```python
from build123d import *

# Parameters (mm, degrees)
SKETCH4_W                = 48.4
SKETCH4_H                = 35.4
BOTTOM_PLATE_DEPTH       = 3
SKETCH5_W                = 48.4
SKETCH5_H                = 3
SKETCH5_H_2              = 3.111627182
SIDE_PLATE_DEPTH         = 32.4
SKETCH6_W                = 48.4
SKETCH6_H                = 3
TOP_PLATE_1_DEPTH        = 6
SKETCH7_W                = 48.4
SKETCH7_H                = 3
TOP_PLATE_2_DEPTH        = 6
CAMERA_SCREW_HOLES_REACH = 64.688
SKETCH8_R                = 1
SKETCH10_R               = 1
CASE_ATTACHMENT_1_DEPTH  = 3
SKETCH10_4_R             = 1
CASE_ATTACHMENT_2_DEPTH  = 3


with BuildPart() as part:
    # Sketch4 → Bottom_Plate (new body)
    with BuildSketch(Plane.XY):
        with Locations((-19.226323529, -13.831389527)):
            Rectangle(SKETCH4_W, SKETCH4_H)
    extrude(amount=BOTTOM_PLATE_DEPTH)

    # Sketch5 → Side_Plate (add)
    with BuildSketch(Plane.XY.offset(3)):
        with Locations((-19.226323529, 2.368610473)):
            Rectangle(SKETCH5_W, SKETCH5_H)
        with Locations((-19.226323529, -29.975575936)):
            Rectangle(SKETCH5_W, SKETCH5_H_2)
    extrude(amount=SIDE_PLATE_DEPTH)

    # Sketch6 → Top_Plate_1 (add)
    with BuildSketch(Plane.XZ.offset(-0.868610473)):
        with Locations((-19.226323529, 33.9)):
            Rectangle(SKETCH6_W, SKETCH6_H)
    extrude(amount=TOP_PLATE_1_DEPTH)

    # Sketch7 → Top_Plate_2 (add)
    with BuildSketch(Plane(origin=(0, -28.419762345, 0), x_dir=(1, 0, 0), z_dir=(0, 1, 0))):
        with Locations((-19.226323529, -33.9)):
            Rectangle(SKETCH7_W, SKETCH7_H)
    extrude(amount=TOP_PLATE_2_DEPTH)

    # Sketch8 → Camera_Screw_Holes (cut, up to next)
    with BuildSketch(Plane.XY.offset(3), mode=Mode.PRIVATE) as camera_screw_holes_sk1:
        with Locations((-34.526323529, -19.719762345)):
            Circle(SKETCH8_R)
    camera_screw_holes_tool1 = extrude(camera_screw_holes_sk1.sketch, amount=-CAMERA_SCREW_HOLES_REACH, mode=Mode.PRIVATE) & part.part
    # Sketch8 → Camera_Screw_Holes (cut, up to next)
    with BuildSketch(Plane.XY.offset(3), mode=Mode.PRIVATE) as camera_screw_holes_sk2:
        with Locations((-34.611878154, -7.831372789)):
            Circle(SKETCH8_R)
    camera_screw_holes_tool2 = extrude(camera_screw_holes_sk2.sketch, amount=-CAMERA_SCREW_HOLES_REACH, mode=Mode.PRIVATE) & part.part
    # Sketch8 → Camera_Screw_Holes (cut, up to next)
    with BuildSketch(Plane.XY.offset(3), mode=Mode.PRIVATE) as camera_screw_holes_sk3:
        with Locations((-12.611878575, -7.835676936)):
            Circle(SKETCH8_R)
    camera_screw_holes_tool3 = extrude(camera_screw_holes_sk3.sketch, amount=-CAMERA_SCREW_HOLES_REACH, mode=Mode.PRIVATE) & part.part
    # Sketch8 → Camera_Screw_Holes (cut, up to next)
    with BuildSketch(Plane.XY.offset(3), mode=Mode.PRIVATE) as camera_screw_holes_sk4:
        with Locations((-12.526323529, -19.719762345)):
            Circle(SKETCH8_R)
    camera_screw_holes_tool4 = extrude(camera_screw_holes_sk4.sketch, amount=-CAMERA_SCREW_HOLES_REACH, mode=Mode.PRIVATE) & part.part
    add(camera_screw_holes_tool1.solids().sort_by_distance((-34.526324, -19.719762, 3))[0], mode=Mode.SUBTRACT)
    add(camera_screw_holes_tool2.solids().sort_by_distance((-34.611878, -7.831373, 3))[0], mode=Mode.SUBTRACT)
    add(camera_screw_holes_tool3.solids().sort_by_distance((-12.611879, -7.835677, 3))[0], mode=Mode.SUBTRACT)
    add(camera_screw_holes_tool4.solids().sort_by_distance((-12.526324, -19.719762, 3))[0], mode=Mode.SUBTRACT)

    # Sketch10 → Case_Attachment_1 (add)
    with BuildSketch(Plane(origin=(0, 0, 0), x_dir=(-1, 0, 0), z_dir=(0, 0, -1))):
        with BuildLine():
            Line((4.226323529, 6.201943806), (4.226323529, 3.868610473))
            Line((4.226323529, 3.868610473), (34.226323529, 3.868610473))
            Line((34.226323529, 3.868610473), (34.226323529, 6.201943806))
            ThreePointArc((34.226323529, 6.201943806), (33.634696523, 8.561233434), (31.99982451, 10.362195278))
            Line((31.99982451, 10.362195278), (21.99982451, 17.028861945))
            ThreePointArc((21.99982451, 17.028861945), (19.226323529, 17.868610473), (16.452822548, 17.028861945))
            Line((16.452822548, 17.028861945), (6.452822548, 10.362195278))
            ThreePointArc((6.452822548, 10.362195278), (4.817950535, 8.561233434), (4.226323529, 6.201943806))
        make_face()
        with Locations((9.226323529, 6.201943806)):
            Circle(SKETCH10_R, mode=Mode.SUBTRACT)
        with Locations((29.226323529, 6.201943806)):
            Circle(SKETCH10_R, mode=Mode.SUBTRACT)
        with Locations((19.226323529, 12.868610473)):
            Circle(SKETCH10_R, mode=Mode.SUBTRACT)
    extrude(amount=-CASE_ATTACHMENT_1_DEPTH)

    # Sketch10<4> → Case_Attachment_2 (add)
    with BuildSketch(Plane(origin=(0, 0, 0), x_dir=(-1, 0, 0), z_dir=(0, 0, -1))):
        with BuildLine():
            ThreePointArc((4.226323529, -33.86472286), (4.817950535, -36.224012488), (6.452822548, -38.024974332))
            Line((6.452822548, -38.024974332), (16.452822548, -44.691640999))
            ThreePointArc((16.452822548, -44.691640999), (19.226323529, -45.531389527), (21.99982451, -44.691640999))
            Line((21.99982451, -44.691640999), (31.99982451, -38.024974332))
            ThreePointArc((31.99982451, -38.024974332), (33.634696523, -36.224012488), (34.226323529, -33.86472286))
            Line((34.226323529, -33.86472286), (34.226323529, -31.531389527))
            Line((34.226323529, -31.531389527), (4.226323529, -31.531389527))
            Line((4.226323529, -31.531389527), (4.226323529, -33.86472286))
        make_face()
        with Locations((9.226323529, -33.86472286)):
            Circle(SKETCH10_4_R, mode=Mode.SUBTRACT)
        with Locations((19.226323529, -40.531389527)):
            Circle(SKETCH10_4_R, mode=Mode.SUBTRACT)
        with Locations((29.226323529, -33.86472286)):
            Circle(SKETCH10_4_R, mode=Mode.SUBTRACT)
    extrude(amount=-CASE_ATTACHMENT_2_DEPTH)


solid = part.part
```
CAD build for the part. Positions are in the model's coordinates, mm. A direction names the side the tool comes from. Give positions to 0.01 mm unless a question says otherwise; leave off trailing zeros. Write each loop counter-clockwise with the first axis right and the second up, starting at its lowest first coordinate (ties: lowest second). Pieces come first, ordered by that corner, then holes. Notation, with made-up numbers: (64, -30.5) -> (91, -30.5) arc R29 cw to (91, -10.5) -> close; hole circle Ø1 at (58, -2.75). An arc over 180 degrees is marked (long way). Write each question's results on one line, items separated by ' | '.
1. Two-plate mould, pull along Z, no slides. Class faces 4 (the flat face through (-20, -27, 35.4)), 5 (the flat face through (-20, 0.869, 17)), 6 (the cylindrical face through (-33.65, 8.53, 1.48)), 7 (the flat face through (-20, -28.42, 17)): pulls with the +Z half, pulls with the -Z half, needs draft (parallel to the pull), parting line crosses it, or undercut.
Geometry check:
face 4: pulls with the +Z half | face 5: undercut | face 6: needs draft | face 7: undercut
2. Wall check: probe 1 along Y at (x, z) = (-19, 23.5); probe 2 along Z at (x, y) = (-16.5, -2.5); probe 3 along Y at (x, z) = (1, 2.5). Give the ranges that are in metal, low to high. Write a range as [from, to].
Geometry check:
probe 1: [-31.53, -28.42], [0.87, 3.87] | probe 2: [0, 3], [32.4, 35.4] | probe 3: [-31.53, 3.87]
3. Drop flat-ended pins along their axis: P1, Ø2.5, axis at x = -12.53, y = -19.72, coming from the +Z side; P2, Ø9, axis at x = -10, z = 14.5, coming from the +Y side; P3, Ø1.5, axis at x = -23, z = 5.5, coming from the -Y side. Give the stop position or say it passes through.
Geometry check:
P1: z = 3 | P2: y = 3.87 | P3: y = -31.53
4. Cut at B-B, the plane x = 2. Write the cut outline in (y, z).
Geometry check:
outline: (-31.53, 0) -> (3.87, 0) -> (3.87, 35.4) -> (-5.13, 35.4) -> (-5.13, 32.4) -> (0.87, 32.4) -> (0.87, 3) -> (-28.42, 3) -> (-28.42, 32.4) -> (-22.42, 32.4) -> (-22.42, 35.4) -> (-31.53, 35.4) -> close
5. Cut at A-A, the plane z = 14. Write the cut outline in (x, y).
Geometry check:
outline: (-43.43, -31.53) -> (4.97, -31.53) -> (4.97, -28.42) -> (-43.43, -28.42) -> close; (-43.43, 0.87) -> (4.97, 0.87) -> (4.97, 3.87) -> (-43.43, 3.87) -> close
6. Cut at C-C, the plane y = -18. Write the cut outline in (x, z).
Geometry check:
outline: (-43.43, 0) -> (4.97, 0) -> (4.97, 3) -> (-43.43, 3) -> close
7. Which spindle directions (+Z, -Z, +X, -X, +Y, -Y) get a long thin tool onto all of the face, cutting with end or side? Do faces 1 (the cylindrical face through (-19.19, -45.53, 1.48)), 2 (the flat face through (-34.226, 5, 1)), 3 (the flat face through (-19, 9, 3)). Say none if no direction does.
Geometry check:
face 1: +Z, -Z, -Y | face 2: +Z, -Z, -X, +Y | face 3: +Z, +X, -X, +Y
